from build123d import *

# Parameters (mm, degrees)
EXTRUDE_THIN1_DEPTH         = 38.1
BOSS_EXTRUDE1_DEPTH         = 2.54
F_3_4_0_75_DIAMETER_HOLE1_D = 19.05
CUT_EXTRUDE1_DEPTH          = 177.53


with BuildPart() as part:
    # Sketch1 → Extrude-Thin1 (new body, symmetric)
    with BuildSketch(Plane(origin=(0, 0, 0), x_dir=(0, 0, -1), z_dir=(1, 0, 0))):
        with BuildLine():
            Line((0, 0), (0, 165.1))
            Line((0, 165.1), (6.35, 176.098522628))
            Line((6.35, 176.098522628), (6.35, 820.325038441))
            Line((6.35, 820.325038441), (142.875, 899.147783942))
            ThreePointArc((142.875, 899.147783942), (167.513381133, 894.246905223), (165.870384182, 869.179615818))
            Line((165.870384182, 869.179615818), (167.666435406, 867.383564594))
            ThreePointArc((167.666435406, 867.383564594), (169.528498617, 895.793159252), (141.605, 901.347488468))
            Line((141.605, 901.347488468), (3.81, 821.791508125))
            Line((3.81, 821.791508125), (3.81, 176.779113577))
            Line((3.81, 176.779113577), (-2.54, 165.780590949))
            Line((-2.54, 165.780590949), (-2.54, 0))
            Line((-2.54, 0), (0, 0))
        make_face()
    extrude(amount=EXTRUDE_THIN1_DEPTH, both=True)

    # Sketch5 → Boss-Extrude1 (add)
    with BuildSketch(Plane(origin=(0, 0, 0), x_dir=(-1, 0, 0), z_dir=(0, 0, -1))):
        Polygon((126.873, 0), (-126.873, 0), (-126.873, 101.6), (-38.1, 165.1), (38.1, 165.1), (126.873, 101.6), align=None)
    extrude(amount=-BOSS_EXTRUDE1_DEPTH)

    # 3/4 (0.75) Diameter Hole1 (through all)
    with Locations(Plane(origin=(0, 0, 0), x_dir=(-1, 0, 0), z_dir=(0, 0, -1))):
        with Locations((0, 19.05), (0, 133.35)):
            Hole(F_3_4_0_75_DIAMETER_HOLE1_D / 2)

    # Sketch4 → Cut-Extrude1 (cut, through all)
    with BuildSketch(Plane.XY.offset(2.54)):
        with BuildLine():
            Line((-3.175, 158.75), (-3.175, 171.45))
            ThreePointArc((-3.175, 171.45), (0, 174.625), (3.175, 171.45))
            Line((3.175, 171.45), (3.175, 158.75))
            ThreePointArc((3.175, 158.75), (0, 155.575), (-3.175, 158.75))
        make_face()
    extrude(amount=-CUT_EXTRUDE1_DEPTH, mode=Mode.SUBTRACT)


solid = part.part
The model under review builds one solid part; all positions refer to its coordinate system, in mm. A direction names the side the tool comes from. Give positions to 0.01 mm unless a question says otherwise; leave off trailing zeros. Order: outer loops, then holes, each group sorted by start corner. A loop starts at its lowest first (then second) coordinate and runs counter-clockwise, first axis right, second up. Notation, with made-up numbers: (63, 54.25) -> (76, 54.25) arc R23 ccw to (76, 89.25) -> close; hole circle Ø3 at (24, 10). An arc over 180 degrees is marked (long way). Write item = value, one per line. Start each with the question number.
(1) Draft analysis for pull direction Y (two halves, no side actions). For faces 5 (the flat face through (1, 494, -6.35)), 6 (the flat face through (-81.87, 133.79, 1.25)), 7 (the cylindrical face through (-1.2, 142.8, 1.3)), 8 (the cylindrical face through (0.533, 895.445, -169.79)), state which applies: +Y half, -Y half, draft (parallel to the pull), parting line (faces both ways), or undercut.
(2) For pin 1 Ø4 at (x, z) = (-28, -43) entering from +Y; pin 2 Ø5 at (y, z) = (167, -1) entering from +X; pin 3 Ø7 at (y, z) = (166, 1) entering from -X, all flat-tipped, find the tip position at first contact; note any pin that passes through.
(3) Take a section at D-D (y = 458). Write out the cut boundary in (x, z), plus the area to 3 significant figures.
(4) Take a section at A-A (y = 19.05). Write out the cut boundary in (x, z) (3 decimals), plus the area to 3 significant figures.
(5) Tool access review of faces 1 (the flat face through (-2, 65, 0)), 2 (the cylindrical face through (0.533, 894.549, -167.277)), 3 (the flat face through (1, 504, -3.81)), 4 (the flat face through (0.533, 859.185, -73.657)): name each direction out of +Z, -Z, +X, -X, +Y, -Y from which nothing blocks a thin tool from reaching the whole face with its end or side.
(6) Take a section at C-C (y = 133.35). Write out the cut boundary in (x, z) (1 decimal), plus the area to 3 significant figures.
(7) For L1, parallel to Y at x = 0, z = 1.25 (3 decimals); L2, parallel to Z at x = -102, y = 90.5; L3, parallel to Z at x = 38, y = 792, list the stretches that pass through material, from the lowest coordinate up. Write a range as from..to.
Returned:
q1.face_5 = draft
q1.face_6 = +Y half
q1.face_7 = undercut
q1.face_8 = parting line
q2.pin_1 = 845.57
q2.pin_2 = 38.65
q2.pin_3 = -41.73
q3.outline = (-38.1, -6.35) -> (38.1, -6.35) -> (38.1, -3.81) -> (-38.1, -3.81) -> close
q3.area = 194 mm²
q4.outline = (-126.873, 0) -> (-9.525, 0) -> (-9.525, 2.54) -> (-126.873, 2.54) -> close; (9.525, 0) -> (126.873, 0) -> (126.873, 2.54) -> (9.525, 2.54) -> close
q4.area = 596 mm²
q5.face_1 = -Z, +X, -X, -Y
q5.face_2 = +X, -X
q5.face_3 = +Z, +X, -X, +Y
q5.face_4 = +X, -X, -Y
q6.outline = (-82.5, 0) -> (-9.5, 0) -> (-9.5, 2.5) -> (-82.5, 2.5) -> close; (9.5, 0) -> (82.5, 0) -> (82.5, 2.5) -> (9.5, 2.5) -> close
q6.area = 371 mm²
q7.L1 = 0..9.525, 28.575..123.825, 142.875..155.575
q7.L2 = 0..2.54
q7.L3 = -6.35..-3.81
